```python
from build123d import *

# Parameters (mm, degrees)
F0_W     = 50.8
F0_H     = 19.05
F1_DEPTH = 774.7
F2_W     = 122.43557321
F2_H     = 50.8
F2_W_2   = 343.1604206562
F2_W_3   = 253.376558423
F3_DEPTH = 25.4
F4_R     = 0.79375
F5_DEPTH = 25.4
F6_R     = 4.7625
F7_DEPTH = 25.4


# Not quite as in the source:
# - a feature names something its author has since deleted; it is built from what else it names


with BuildPart() as f1:
    # F0 (on Top) → F1 (new body)
    with BuildSketch(Plane.XY):
        Rectangle(F0_W, F0_H)
    extrude(amount=F1_DEPTH)

    # F2 (on Front) → F3 (cut)
    with BuildSketch(Plane.XZ):
        with Locations((22.4465244144, 25.4)):
            Rectangle(F2_W, F2_H)
        with Locations((-38.7818217278, 749.3)):
            Rectangle(F2_W_2, F2_H)
        with Locations((-33.7835475802, 647.7)):
            Rectangle(F2_W_3, F2_H)
    extrude(amount=F3_DEPTH, mode=Mode.SUBTRACT)

    # F4 (on Front) → F5 (cut)
    with BuildSketch(Plane.XZ):
        with Locations((9.525, 101.6)):
            Circle(F4_R)
        with Locations((9.525, 155.575)):
            Circle(F4_R)
        with Locations((9.525, 619.125)):
            Circle(F4_R)
        with Locations((9.525, 673.1)):
            Circle(F4_R)
        with Locations((-9.525, 619.125)):
            Circle(F4_R)
        with Locations((-9.525, 673.1)):
            Circle(F4_R)
        with Locations((-9.525, 101.6)):
            Circle(F4_R)
        with Locations((-9.525, 155.575)):
            Circle(F4_R)
    extrude(amount=-F5_DEPTH, mode=Mode.SUBTRACT)

    # F6 (on Front) → F7 (cut)
    with BuildSketch(Plane.XZ):
        with Locations((0, 95.25)):
            Circle(F6_R)
        with Locations((0, 361.95)):
            Circle(F6_R)
    extrude(amount=F7_DEPTH, mode=Mode.SUBTRACT)


solid = f1.part
```
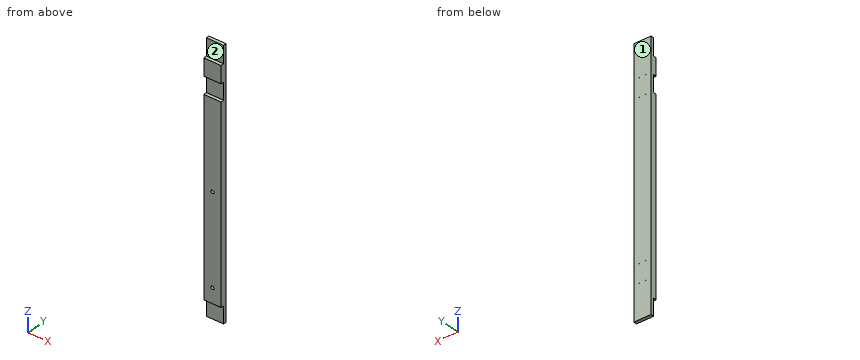
The listing builds one solid part. Answer for the finished solid, in the listing's coordinates (mm). Face numbers are marked on the shaded views. A direction names the side the tool comes from. Coordinates: 2 decimals unless noted, no trailing zeros. Answer as a JSON object with one key per item and string values. Group by question number.
Item 1: Section A-A (y = -4.75) is taken. Give the number of separate pieces and of enclosed holes in the cut face, and give its area (3 significant figures).
Item 2: Consider L1, parallel to X at y = 4.25, z = 673.1; L2, parallel to Z at x = 12.5, y = -1.75; L3, parallel to X at y = -6.75, z = 95.25. Determine where each line is inside the solid, lowest interval first.
Item 3: Each of these flat-tipped pins is pushed along its axis until it touches: P1, Ø0.5, axis at x = -9.5, z = 101.5, coming from the +Y side; P2, Ø3, axis at x = -1.5, y = -3.5, coming from the -Z side; P3, Ø15, axis at x = 9.5, z = 653, coming from the -Y side. Where does it stop, or does it pass through?
Item 4: Which of the six approach directions +Z, -Z, +X, -X, +Y, -Y give full straight-line access (tool end or side, diameter ignored) to the marked faces 1 and 2?
Solved:
{
 "1": {"separate pieces": "2", "enclosed holes": "2", "area": "31,500 mm2"},
 "2": {"L1": "x = -25.4 to -10.32, -8.73 to 8.73, 10.32 to 25.4", "L2": "z = 50.8 to 622.3, 673.1 to 723.9", "L3": "x = -25.4 to -4.76, 4.76 to 25.4"},
 "3": {"P1": "stops at y = 0", "P2": "stops at z = 50.8", "P3": "stops at y = 0"},
 "4": {"face 1": "+Z, -Z, +X, -X, +Y", "face 2": "+Z, +X, -X, -Y"}
}
